Autodesk Fusion 360 part; units mm, degrees
sketch "baseplate" plane through (0, 0, 0) normal (0, 1, 0) x (1, 0, 0)
  line L0 (0, 0) -> (80, 0)
  line L1 (80, 0) -> (80, -40)
  line L2 (80, -40) -> (0, -40)
  line L3 (0, -40) -> (0, 0)
  dimension "d1" = 80
  dimension "d2" = 40
sketch "pryamid_base" plane through (0, 0, 0) normal (0, 1, 0) x (1, 0, 0)
  line L0 (5, -35) -> (15, -35)
  line L1 (15, -35) -> (15, -25)
  line L2 (15, -25) -> (5, -25)
  line L3 (5, -25) -> (5, -35)
  line L4 (35, -35) -> (35, -25)
  line L5 (35, -25) -> (25, -25)
  line L6 (25, -35) -> (35, -35)
  line L7 (25, -25) -> (25, -35)
  line L8 (35, -5) -> (25, -5)
  line L9 (35, -15) -> (35, -5)
  line L10 (15, -5) -> (5, -5)
  line L11 (25, -5) -> (25, -15)
  line L12 (5, -5) -> (5, -15)
  line L13 (5, -15) -> (15, -15)
  line L14 (15, -15) -> (15, -5)
  line L15 (25, -15) -> (35, -15)
  line L16 (55, -15) -> (65, -25)
  circle A0 centre (60, -20) radius 15
  dimension "d3" = 10
  dimension "d4" = 10
  dimension "d5" = 10
  dimension "d6" = 10
  dimension "d11" = 10
  dimension "d12" = 10
  dimension "d13" = 10
  dimension "d14" = 10
  dimension "d48" = 30
ref_plane "WorkPlane1" through (0, 4.5, 0) normal (0, 1, 0) x (0, 0, 1)
sketch "pryamid_offsetplane" plane through (0, 4.5, 0) normal (0, 1, 0) x (1, 0, 0)
  line L0 (7.5, -32.5) -> (12.5, -32.5)
  line L1 (12.5, -32.5) -> (12.5, -27.5)
  line L2 (12.5, -27.5) -> (7.5, -27.5)
  line L3 (7.5, -27.5) -> (7.5, -32.5)
  line L4 (27.5, -27.5) -> (27.5, -32.5)
  line L5 (32.5, -32.5) -> (32.5, -27.5)
  line L6 (27.5, -32.5) -> (32.5, -32.5)
  line L7 (32.5, -27.5) -> (27.5, -27.5)
  line L8 (7.5, -27.5) -> (7.5, -32.5)
  line L9 (12.5, -32.5) -> (12.5, -27.5)
  line L10 (7.5, -32.5) -> (12.5, -32.5)
  line L11 (12.5, -27.5) -> (7.5, -27.5)
  line L12 (27.5, -7.5) -> (27.5, -12.5)
  line L13 (12.5, -12.5) -> (12.5, -7.5)
  line L14 (12.5, -7.5) -> (7.5, -7.5)
  line L15 (7.5, -7.5) -> (7.5, -12.5)
  line L16 (7.5, -12.5) -> (12.5, -12.5)
  line L17 (32.5, -7.5) -> (27.5, -7.5)
  line L18 (27.5, -12.5) -> (32.5, -12.5)
  line L19 (12.5, -7.5) -> (7.5, -7.5)
  line L20 (32.5, -12.5) -> (32.5, -7.5)
  line L21 (12.5, -12.5) -> (12.5, -7.5)
  line L22 (7.5, -12.5) -> (12.5, -12.5)
  line L23 (7.5, -7.5) -> (7.5, -12.5)
  circle A0 centre (60, -20) radius 12.5
  dimension "d49" = 25
extrude "Extrude1" add sketch "baseplate" against normal blind 5
loft "Loft1" add profiles "pryamid_base", "pryamid_offsetplane" section 1 contours L0 L1 L2 L3 section 2 contours L0 L1 L2 L3 L8 L9 L10 L11
loft "Loft2" add profiles "pryamid_base", "pryamid_offsetplane" section 1 contours L4 L5 L6 L7 section 2 contours L4 L5 L6 L7
sketch "sidewall" plane through (0, 0, 0) normal (0, 1, 0) x (1, 0, 0)
  line L0 (0, 0) -> (-8, 0)
  line L1 (-8, 0) -> (-8, -40)
  line L2 (-8, -40) -> (0, -40)
  line L3 (0, -40) -> (0, 0)
  dimension "d22" = 8
extrude "Extrude2" add sketch "sidewall" along normal blind 40 and the other way blind 5
sketch "sidemount" plane through (0, 0, 0) normal (0, 1, 0) x (1, 0, 0)
  line L0 (80, 0) -> (88, 0)
  line L1 (88, 0) -> (88, -40)
  line L2 (88, -40) -> (80, -40)
  line L3 (80, -40) -> (80, 0)
extrude "Extrude3" add sketch "sidemount" against normal blind 5
sketch "holes" plane through (0, -5, 0) normal (0, -1, 0) x (1, 0, 0)
  line L0 (88, 40) -> (-8, 40)
  line L1 (-8, 40) -> (-8, 0)
  line L2 (-8, 0) -> (88, 0)
  line L3 (88, 0) -> (88, 40)
  line L4 (-8, 0) -> (-4, 0)
  line L5 (-8, 6) -> (-8, 0)
  line L6 (-4, 40) -> (-8, 40)
  line L7 (-8, 40) -> (-8, 34)
  circle A0 centre (-4, 34) radius 2
  circle A1 centre (-4, 6) radius 2
  circle A2 centre (-4, 34) radius 3.4
  circle A3 centre (-4, 6) radius 3.4
  dimension "d29" = 6
  dimension "d30" = 4
  dimension "d31" = 4
  dimension "d32" = 6.8
  dimension "d33" = 6.8
extrude "Extrude4" cut sketch "holes" against normal blind 51 contours A0 | A1
extrude "Extrude5" cut sketch "holes" against normal blind 5 contours A2 | A3
sketch "holes (1)" plane through (0, -5, 0) normal (0, -1, 0) x (1, 0, 0)
  circle A0 centre (84, 34) radius 2
  circle A1 centre (84, 6) radius 2
  circle A2 centre (84, 34) radius 3.4
  circle A3 centre (84, 6) radius 3.4
  dimension "d42" = 4
  dimension "d43" = 4
  dimension "d44" = 6.8
  dimension "d45" = 6.8
extrude "Extrude6" cut sketch "holes (1)" against normal blind 16 contours A0 | A1
loft "Loft9" add profiles "pryamid_offsetplane", "pryamid_base" section 1 contours L13 L14 L15 L16 L19 L21 L22 L23 section 2 contours L10 L12 L13 L14
loft "Loft10" add profiles "pryamid_base", "pryamid_offsetplane" section 1 contours L8 L9 L11 L15 section 2 contours L12 L17 L18 L20
loft "Loft11" add profiles "pryamid_offsetplane", "pryamid_base" section 1 contours A0 section 2 contours A0
Input: part model. Units: mm. Frame: model coordinates. A direction names the side the tool comes from. Coordinates: 2 decimals unless noted, no trailing zeros. Loops run counter-clockwise (first coordinate to the right, second up) from the corner with the lowest first, then second, coordinate; pieces in that order, holes last.
Q1. Draft query along Z for faces 1 (the face through (-0.757, -2.535, 7.021)), 2 (the face through (88, -2, 20)), 3 (the face through (22, -1, 0)), 4 (the face through (-4, 20, 32)). Return one class per face: +Z half, -Z half, draft (parallel to the pull), parting line (faces both ways), or undercut.
Q2. Material intervals for line 1 (Z direction, x = -4, y = 9); line 2 (Z direction, x = -4, y = -1.55); line 3 (Y direction, x = 38, z = 7), sorted ascending.
Q3. Cut plane B-B (y = 33.5). Output: boundary loops of the cut face in (x, z), then the cut area to 3 significant figures.
Q4. Cut plane C-C (x = -4). Output: boundary loops of the cut face in (y, z).
Q5. Set-up query: faces 5 (the face through (-0.86, -2.54, 32.7)), 6 (the face through (43, 0, 20)), 7 (the face through (60, 4.5, 20)). Return all of +Z, -Z, +X, -X, +Y, -Y with unobstructed straight access to the full face (end or side cutting, diameter ignored); none if empty.
Q6. Cut plane D-D (x = 18.5). Output: boundary loops of the cut face in (y, z), then the cut area to 3 significant figures.
Q7. Contact query for flat-ended pins moving along their axis: pin 1 (5 mm diameter, centred on x = -4, z = 6, fed in from +Y); pin 2 (1.5 mm diameter, centred on x = 30.5, z = 31, fed in from +Y); pin 3 (6.5 mm diameter, centred on x = 84, z = 34, fed in from +Y); pin 4 (4.5 mm diameter, centred on x = -4, z = 34, fed in from -Y). Output: stop coordinate, or through.
Q8. Cut plane A-A (x = 84). Output: boundary loops of the cut face in (y, z).
Working result:
1. face 1: undercut
1. face 2: draft
1. face 3: -Z half
1. face 4: undercut
2. line 1: z = 0 to 4, 8 to 32, 36 to 40
2. line 2: z = 0 to 2.6, 9.4 to 30.6, 37.4 to 40
2. line 3: y = -5 to 0
3. outline: (-8, 0) - (0, 0) - (0, 40) - (-8, 40) - close; hole circle Ø4 at (-4, 6); hole circle Ø4 at (-4, 34)
3. area: 295 mm2
4. outline: (-5, 0) - (40, 0) - (40, 4) - (0, 4) - (0, 2.6) - (-5, 2.6) - close; (-5, 9.4) - (0, 9.4) - (0, 8) - (40, 8) - (40, 32) - (0, 32) - (0, 30.6) - (-5, 30.6) - close; (-5, 37.4) - (0, 37.4) - (0, 36) - (40, 36) - (40, 40) - (-5, 40) - close
5. face 5: -Y
5. face 6: +Y
5. face 7: +Z, -Z, +X, +Y
6. outline: (-5, 0) - (0, 0) - (0, 40) - (-5, 40) - close
6. area: 200 mm2
7. pin 1: stops at y = 40
7. pin 2: stops at y = 4.5
7. pin 3: stops at y = 0
7. pin 4: stops at y = 0
8. outline: (-5, 0) - (0, 0) - (0, 4) - (-5, 4) - close; (-5, 8) - (0, 8) - (0, 32) - (-5, 32) - close; (-5, 36) - (0, 36) - (0, 40) - (-5, 40) - close
